Part model, mm, in its own coordinate system. A direction names the side the tool comes from. Round coordinates to 2 decimals unless told otherwise and drop trailing zeros. Write each loop counter-clockwise with the first axis right and the second up, starting at its lowest first coordinate (ties: lowest second). Pieces come first, ordered by that corner, then holes.
```python
from build123d import *

# Parameters (mm, degrees)
F0_W     = 304.8
F0_H     = 152.4
F1_DEPTH = 88.9
F2_T     = -2.54


with BuildPart() as f1:
    # F0 (on Front) → F1 (new body, symmetric)
    with BuildSketch(Plane.XZ):
        with Locations((-43.711439, -5.892325)):
            Rectangle(F0_W, F0_H)
    extrude(amount=F1_DEPTH, both=True)

    # F2
    f2_openings = [f1.faces().sort_by_distance(p)[0] for p in [
        (-43.711439, -88.9, -5.892325),
        (-196.111439, 0, -5.892325),
        (108.688561, 0, -5.892325),
    ]]
    offset(amount=F2_T, openings=f2_openings)


solid = f1.part
```
Q1. Cut at A-A on y = 63.5. Write the cut outline in (x, z), plus the area to 3 significant figures.
Values follow:
outline: (-196.11, -82.09) - (108.69, -82.09) - (108.69, -79.55) - (-196.11, -79.55) - close; (-196.11, 67.77) - (108.69, 67.77) - (108.69, 70.31) - (-196.11, 70.31) - close
area: 1,550 mm2
Q2. Which spindle directions (+Z, -Z, +X, -X, +Y, -Y) get a long thin tool onto all of the face, cutting with end or side? Do faces 1 (the flat face through (-46, -2, 67.768)), 2 (the flat face through (-46, -1, 70.308)). Say none if no direction does.
Values follow:
face 1: +X, -X, -Y
face 2: +Z, +X, -X, +Y, -Y
Q3. Mould opens along Z. For faces 3 (the flat face through (-196.111, 0, -80)), 4 (the flat face through (-46, -2, -79.552)), 5 (the flat face through (-46, -1, -82.092)) say: +Z half, -Z half, draft (parallel to the pull), parting line (faces both ways), or undercut.
Values follow:
face 3: draft
face 4: undercut
face 5: -Z half
Q4. Wall check: L1, parallel to Z at x = -165, y = 81.5; L2, parallel to Y at x = -160, z = 26.5. Give the ranges that are in metal, low to high.
Values follow:
L1: z = -82.09 to -79.55, 67.77 to 70.31
L2: y = 86.36 to 88.9
Q5. Cut at B-B on x = -141.5. Write the cut outline in (y, z).
Values follow:
outline: (-88.9, -82.09) - (88.9, -82.09) - (88.9, 70.31) - (-88.9, 70.31) - (-88.9, 67.77) - (86.36, 67.77) - (86.36, -79.55) - (-88.9, -79.55) - close
Q6. Cut at C-C on z = -66. Write the cut outline in (x, y), plus the area to 3 significant figures.
Values follow:
outline: (-196.11, 86.36) - (108.69, 86.36) - (108.69, 88.9) - (-196.11, 88.9) - close
area: 774 mm2
